Autodesk Inventor part; units mm, degrees
ref_plane "YZ Plane" through (0, 0, 0) normal (1, 0, 0) x (0, 1, 0)
ref_plane "XZ Plane" through (0, 0, 0) normal (0, 1, 0) x (-1, 0, 0)
ref_plane "XY Plane" through (0, 0, 0) normal (0, 0, 1) x (1, 0, 0)
sketch "Sketch1" plane through (0, 0, 0) normal (0, 0, 1) x (1, 0, 0)
  circle A0 centre (0, 0) radius 7.62
  dimension "d0" = 15.24
extrude "Extrusion1" add sketch "Sketch1" along normal blind 5.08
chamfer "Chamfer1" distance 1.27 angle 45 1 edges at (-7.62, 0, 5.08)
fillet "Fillet1" radius 3.81 1 edges at (-6.35, 0, 5.08)
sketch "Sketch2" plane through (0, 0, 5.08) normal (0, 0, 1) x (1, 0, 0)
  line L0 (-0.7017, 1.8442) -> (0.7248, 1.8442) construction
  line L1 (0.7248, 1.8442) -> (0.7248, -1.2038) construction
  line L2 (0.7248, -1.2038) -> (-0.7017, -1.2038) construction
  line L3 (-0.7017, -1.2038) -> (-0.7017, 1.8442) construction
  line L4 (-0.704, -1.2038) -> (-0.1186, 1.8442)
  line L5 (-0.1186, 1.8442) -> (0.0975, 1.8442)
  line L6 (0.0975, 1.8442) -> (0.7224, -1.2038)
  line L7 (0.7224, -1.2038) -> (0.4924, -1.2038)
  line L8 (0.4924, -1.2038) -> (0.3159, -0.2815)
  line L9 (0.3159, -0.2815) -> (-0.3253, -0.2815)
  line L10 (-0.3253, -0.2815) -> (-0.4903, -1.2038)
  line L11 (-0.4903, -1.2038) -> (-0.704, -1.2038)
  line L12 (-0.2649, 0.0461) -> (0.2531, 0.0461)
  line L13 (0.2531, 0.0461) -> (0.0952, 0.8917)
  spline S0 degree 2 poles (0.0952, 0.8917) (0.0208, 1.2774) (-0.014, 1.5236) knots 0 0 0 1 1 1
  spline S1 degree 2 poles (-0.014, 1.5236) (-0.0442, 1.2309) (-0.0976, 0.9428) knots 0 0 0 1 1 1
  line L14 (-0.0976, 0.9428) -> (-0.2649, 0.0461)
extrude "Extrusion2" cut sketch "Sketch2" against normal blind 0.0635
properties part number "A Button"
Here's how the part is built. I have some questions about the finished solid (model axes, mm). Give positions to 0.01 mm unless a question says otherwise; leave off trailing zeros. Order: outer loops, then holes, each group sorted by start corner. A loop starts at its lowest first (then second) coordinate and runs counter-clockwise, first axis right, second up. Notation, with made-up numbers: M -7,-33.5 L 34,-33.5 A21 ccw 34,-27.5 Z; hole C -23,-18 d4. An arc over 180 degrees is marked long. Use a Markdown table: item, result. Add a question column.
1. For pin 1 Ø3 at (y, z) = (2, 1.5) entering from +X; pin 2 Ø3 at (y, z) = (2.5, 2) entering from -X, each with a flat end and sliding along its axis, tell me the tip position at first contact or that it passes through.
2. Suppose I cut it at B-B (z = 4.2). List the corners of the cut face in (x, y) for me.
3. Suppose I cut it at A-A (z = 0.75). List the corners of the cut face in (x, y) for me.
4. I need wall thicknesses on probe 1 along X at (y, z) = (0.25, 3.7); probe 2 along X at (y, z) = (1.5, 0.4). Which ranges of each line are inside material? Lowest first, please. Write a range as from..to.
5. If we mould it in two halves opening along X, with no side actions, what happens to faces 1 (the flat face through (0, -1, 5.08)), 2 (the flat face through (0.11, -0.12, 5.016)), 3 (the cylindrical face through (-1.65, 7.44, 1.88))? For each: +X half, -X half, draft (parallel to the pull), parting line (faces both ways), or undercut.
Results list:
| question | item | result |
|---|---|---|
| 1 | pin 1 | stops at x = 7.6 |
| 1 | pin 2 | stops at x = -7.55 |
| 2 | outline | C 0,0 d14.41 |
| 3 | outline | C 0,0 d15.24 |
| 4 | probe 1 | x = -7.62..7.62 |
| 4 | probe 2 | x = -7.47..7.47 |
| 5 | face 1 | draft |
| 5 | face 2 | undercut |
| 5 | face 3 | parting line |
